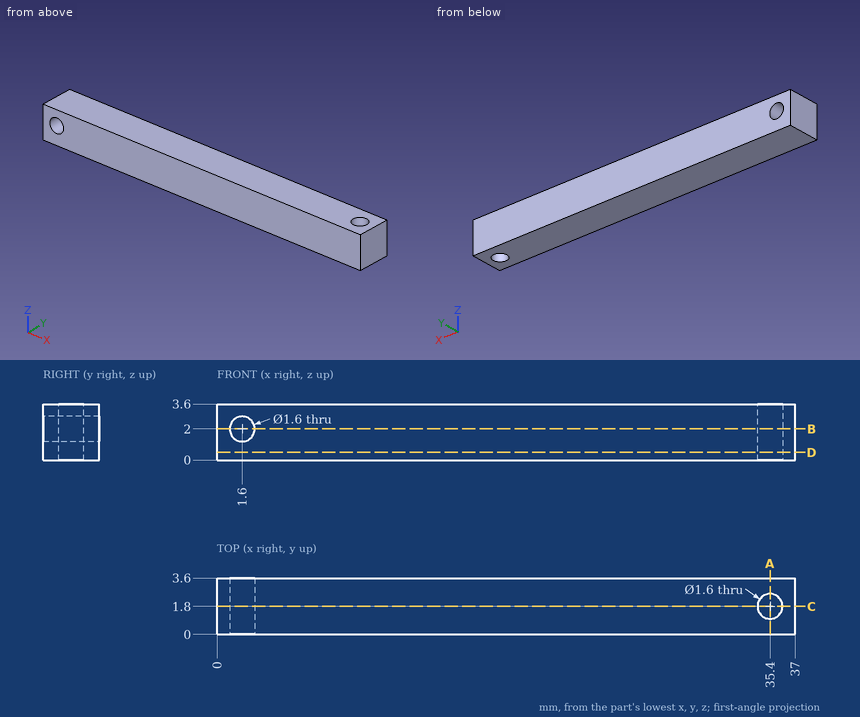
Input: dimensioned drawing with shaded views. Units: mm. Origin: part minimum x, y, z. Give positions to 0.01 mm unless a question says otherwise; leave off trailing zeros. Write each loop counter-clockwise with the first axis right and the second up, starting at its lowest first coordinate (ties: lowest second). Pieces come first, ordered by that corner, then holes.
1. Section query B-B, the plane z = 2. Return loops of the section in (x, y), then the cut area to 3 significant figures.
2. Section query D-D, the plane z = 0.5. Return loops of the section in (x, y).
3. Line query: probe 1 along X at (y, z) = (1.95, 1.4); probe 2 along X at (y, z) = (2, 1.8); probe 3 along Y at (x, z) = (35.4, 1). Output: solid intervals per line, ascending.
4. Section query C-C, the plane y = 1.8. Return loops of the section in (x, z), then the cut area to 3 significant figures.
5. Section query A-A, the plane x = 35.4. Return loops of the section in (y, z), then the cut area to 3 significant figures.
Computed:
1. outline: (0, 0) - (0.8, 0) - (0.8, 3.6) - (0, 3.6) - close; (2.4, 0) - (37, 0) - (37, 3.6) - (2.4, 3.6) - close; hole circle Ø1.6 at (35.4, 1.8)
1. area: 125 mm2
2. outline: (0, 0) - (37, 0) - (37, 3.6) - (0, 3.6) - close; hole circle Ø1.6 at (35.4, 1.8)
3. probe 1: x = 0 to 1.07, 2.13 to 34.61, 36.19 to 37
3. probe 2: x = 0 to 0.83, 2.37 to 34.63, 36.17 to 37
3. probe 3: y = 0 to 1, 2.6 to 3.6
4. outline: (0, 0) - (34.6, 0) - (34.6, 3.6) - (0, 3.6) - close; (36.2, 0) - (37, 0) - (37, 3.6) - (36.2, 3.6) - close; hole circle Ø1.6 at (1.6, 2)
4. area: 125 mm2
5. outline: (0, 0) - (1, 0) - (1, 3.6) - (0, 3.6) - close; (2.6, 0) - (3.6, 0) - (3.6, 3.6) - (2.6, 3.6) - close
5. area: 7.20 mm2
